```python
from build123d import *

# Parameters (mm, degrees)
F1_DEPTH  = 41
F2_R      = 16.3
F3_DEPTH  = 6
F5_DEPTH  = 6.25
F6_R      = 16
F7_DEPTH  = 10.75
F8_R      = 15
F9_DEPTH  = 4
F10_R     = 16.35
F11_DEPTH = 6.8
F12_R     = 13.65
F13_DEPTH = 2
F14_R     = 6
F15_DEPTH = 72.801
F16_R     = 2.85
F17_DEPTH = 26
F21_R     = 3
F22_DEPTH = 45
F23_SIZE  = 6
F24_R     = 2.85
F25_DEPTH = 72.8010001


with BuildPart() as f1:
    # F0 (on Front) → F1 (new body)
    with BuildSketch(Plane.XZ):
        Polygon((0, -20.7846096908), (18, -10.3923048454), (18, 10.3923048454), (0, 20.7846096908), (-18, 10.3923048454), (-18, -10.3923048454), align=None)
    extrude(amount=-F1_DEPTH)

    # F2 (on face) → F3 (join)
    with BuildSketch(Plane(origin=(0, 41, 0), x_dir=(-1, 0, 0), z_dir=(0, 1, 0))):
        Circle(F2_R)
    extrude(amount=F3_DEPTH)

    # F4 (on face) → F5 (join)
    with BuildSketch(Plane(origin=(0, 47, 0), x_dir=(-1, 0, 0), z_dir=(0, 1, 0))):
        Polygon((0, -20.7846096908), (18, -10.3923048454), (18, 10.3923048454), (0, 20.7846096908), (-18, 10.3923048454), (-18, -10.3923048454), align=None)
    extrude(amount=F5_DEPTH)

    # F6 (on face) → F7 (join)
    with BuildSketch(Plane(origin=(0, 53.25, 0), x_dir=(-1, 0, 0), z_dir=(0, 1, 0))):
        Circle(F6_R)
    extrude(amount=F7_DEPTH)

    # F8 (on face) → F9 (join)
    with BuildSketch(Plane(origin=(0, 64, 0), x_dir=(-1, 0, 0), z_dir=(0, 1, 0))):
        Circle(F8_R)
    extrude(amount=F9_DEPTH)

    # F10 (on face) → F11 (join)
    with BuildSketch(Plane(origin=(0, 68, 0), x_dir=(-1, 0, 0), z_dir=(0, 1, 0))):
        Circle(F10_R)
    extrude(amount=F11_DEPTH)

    # F12 (on face) → F13 (cut)
    with BuildSketch(Plane(origin=(0, 74.8, 0), x_dir=(-1, 0, 0), z_dir=(0, 1, 0))):
        Circle(F12_R)
    extrude(amount=-F13_DEPTH, mode=Mode.SUBTRACT)

    # F14 (on face) → F15 (cut, through all)
    with BuildSketch(Plane(origin=(0, 72.8, 0), x_dir=(-1, 0, 0), z_dir=(0, 1, 0))):
        with Locations((5, 0)):
            Circle(F14_R)
    extrude(amount=-F15_DEPTH, mode=Mode.SUBTRACT)

    # F16 (on face) → F17 (cut)
    with BuildSketch(Plane(origin=(0, 72.8, 0), x_dir=(-1, 0, 0), z_dir=(0, 1, 0))):
        with Locations((-4.87, -6.95)):
            Circle(F16_R)
        with Locations((-8.5, 0)):
            Circle(F16_R)
    extrude(amount=-F17_DEPTH, mode=Mode.SUBTRACT)

    # F19 (on offset) → F20 (revolve, cut)
    with BuildSketch(Plane.XZ.offset(-44)):
        Polygon((19.0103325466, 10.8889942077), (15.2210576437, 12.8681406677), (4.87, -6.95), (8.6592749029, -8.9291464601), align=None)
    revolve(axis=Axis((11.6872206375, 44, 6.1022543886), (0.4629582363, 0, 0.8863800942)), mode=Mode.SUBTRACT)

    # F21 (on face) → F22 (cut)
    with BuildSketch(Plane.XZ):
        with Locations((13.4, 7.7364936071)):
            Circle(F21_R)
    extrude(amount=-F22_DEPTH, mode=Mode.SUBTRACT)

    # F23
    f23_edges = [f1.edges().sort_by_distance(p)[0] for p in [
        (-18, 0, 0),
    ]]
    chamfer(f23_edges, length=F23_SIZE)

    # F24 (on face) → F25 (cut, through all)
    with BuildSketch(Plane(origin=(0, 72.8, 0), x_dir=(-1, 0, 0), z_dir=(0, 1, 0))):
        with Locations((-4.62, 7.15)):
            Circle(F24_R)
    extrude(amount=-F25_DEPTH, mode=Mode.SUBTRACT)


solid = f1.part
```
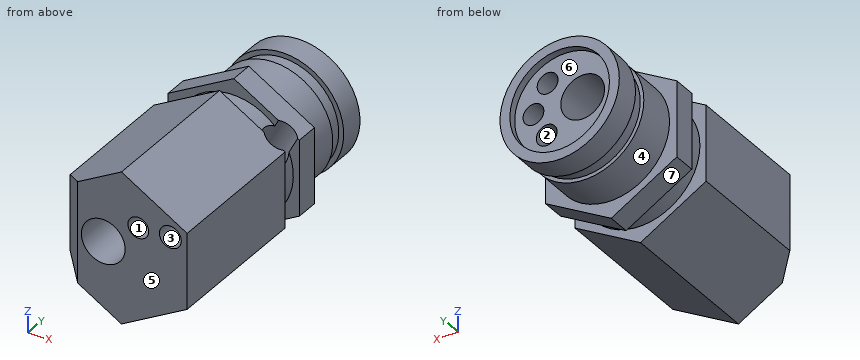
Geometry check sheet. Reference: the model listing, model coordinates, mm. Face numbers are marked on the shaded views. A direction names the side the tool comes from. Coordinates: 2 decimals unless noted, no trailing zeros. Order: outer loops, then holes, each group sorted by start corner. A loop starts at its lowest first (then second) coordinate and runs counter-clockwise, first axis right, second up. Notation, with made-up numbers: M -7,87 L 8,87 A36 cw 8,126 Z; hole C 11,-16 d6. An arc over 180 degrees is marked long. Answer as a JSON object with one key per item and string values.
Q1. Cross-section at B-B on y = 10. Record the cut outline in (x, z).
Results are:
{"outline": "M -18,-10.39 L 0,-20.78 L 18,-10.39 L 18,10.39 L 0,20.78 L -18,10.39 Z; hole C -5,0 d12; hole C 4.62,7.15 d5.7; hole C 13.4,7.74 d6"}
Q2. Release check for a two-part mould opening along X. For the marked faces 5, 6 and 7 record: released by +X, released by -X, zero draft, split by the parting line, or undercut.
Results are:
{"face 5": "zero draft", "face 6": "undercut", "face 7": "released by -X"}
Q3. Tool access check on the marked faces 1, 2, 3 and 4. Record the directions out of +Z, -Z, +X, -X, +Y, -Y that give a thin tool (end or side, any length) a straight path to the whole face; none if there is none.
Results are:
{"face 1": "+Y, -Y", "face 2": "+Y", "face 3": "-Y", "face 4": "none"}
Q4. Depth check by flat-ended pin: pin 1 Ø6.5 at (x, z) = (8.5, 0) entering from +Y; pin 2 Ø2 at (x, y) = (-12.5, 28) entering from +Z; pin 3 Ø1 at (y, z) = (63.5, 4) entering from +X. Enter the tip coordinate at first touch or a pass-through.
Results are:
{"pin 1": "stops at y = 72.8", "pin 2": "stops at z = 14.15", "pin 3": "stops at x = 15.61"}
Q5. Scan lines: line 1 (Y direction, x = -11.5, z = 10); line 2 (Y direction, x = 3.5, z = 16); line 3 (X direction, y = 53, z = 7.15). Record each from-to range of solid material in increasing order.
Results are:
{"line 1": "y = 0 to 64, 68 to 74.8", "line 2": "y = 0 to 41, 47 to 53.25", "line 3": "x = -18 to 1.77, 7.47 to 18"}
